Answer from the drawing. Dimensions are ordinates in mm from the lowest x, y and z of the part. A direction names the side the tool comes from. Coordinates: 2 decimals unless noted, no trailing zeros. Loops run counter-clockwise (first coordinate to the right, second up) from the corner with the lowest first, then second, coordinate; pieces in that order, holes last. Notation, with made-up numbers: (-34.5, 41.25) -> (-5.5, 41.25) arc R23 cw to (-5.5, 66.25) -> close; hole circle Ø4 at (28, 83.25). An arc over 180 degrees is marked (long way). Use a Markdown table: item, result.
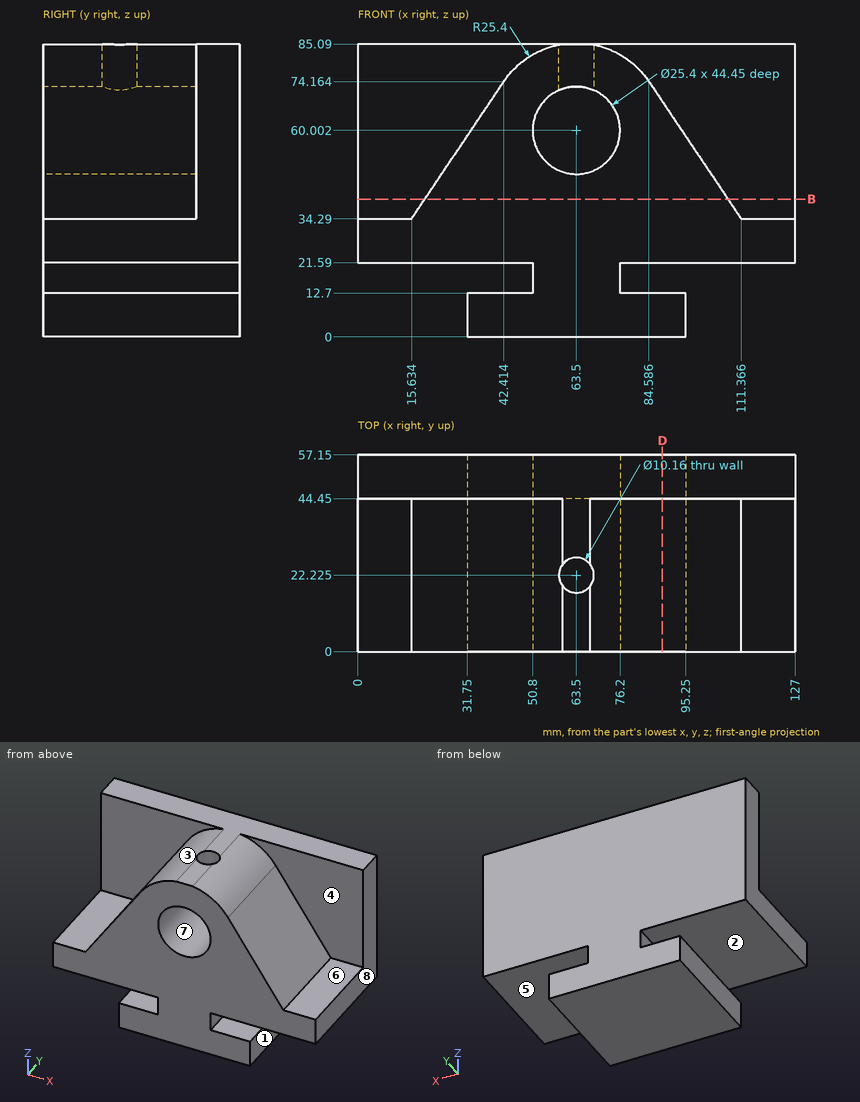
Q1. Section D-D on x = 88.5 is taken. Determine the outline of the cut face in (y, z), and give its area (3 significant figures).
Solved:
| item | result |
|---|---|
| outline | (0, 0) -> (57.15, 0) -> (57.15, 12.7) -> (0, 12.7) -> close; (0, 21.59) -> (57.15, 21.59) -> (57.15, 85.09) -> (44.45, 85.09) -> (44.45, 68.34) -> (0, 68.34) -> close |
| area | 3,610 mm² |
Q2. Determine the mould class of the marked faces 5, 6, 7 and 8 for opening direction Z: pulls with the +Z half, pulls with the -Z half, needs draft (parallel to the pull), parting line crosses it, or undercut.
Solved:
| item | result |
|---|---|
| face 5 | undercut |
| face 6 | pulls with the +Z half |
| face 7 | undercut |
| face 8 | needs draft |
Q3. Section B-B on z = 40 is taken. Determine the outline of the cut face in (x, y), and give its area (3 significant figures).
Solved:
| item | result |
|---|---|
| outline | (0, 44.45) -> (19.47, 44.45) -> (19.47, 0) -> (107.53, 0) -> (107.53, 44.45) -> (127, 44.45) -> (127, 57.15) -> (0, 57.15) -> close |
| area | 5,530 mm² |
Q4. Given pin 1 Ø8 at (x, y) = (63.5, 22.225) entering from +Z; pin 2 Ø4.5 at (x, y) = (123, 31.5) entering from +Z; pin 3 Ø1 at (x, z) = (65, 68.5) entering from -Y; pin 4 Ø15 at (x, z) = (31, 63) entering from -Y, each flat-ended and moving along its own axis, determine where each tip first touches the part or whether it passes through.
Solved:
| item | result |
|---|---|
| pin 1 | z = 47.95 |
| pin 2 | z = 34.29 |
| pin 3 | y = 44.45 |
| pin 4 | y = 0 |
Q5. Consider line 1 (Z direction, x = 40.5, y = 51); line 2 (Z direction, x = 63.5, y = 11); line 3 (X direction, y = 9, z = 19). Determine where each line is inside the solid, lowest interval first. Write a range as [from, to].
Solved:
| item | result |
|---|---|
| line 1 | [0, 12.7], [21.59, 85.09] |
| line 2 | [0, 47.3], [72.7, 85.09] |
| line 3 | [50.8, 76.2] |
Q6. For the marked faces 1, 2, 3 and 4, determine the directions among +Z, -Z, +X, -X, +Y, -Y from which every point of the face is accessible in a straight line to the end or side of a thin tool.
Solved:
| item | result |
|---|---|
| face 1 | -Z, +X, +Y, -Y |
| face 2 | -X, +Y, -Y |
| face 3 | +Z, -X, -Y |
| face 4 | +Z, +X, -Y |
